```python
from build123d import *

# Parameters (mm, degrees)
F1_DEPTH     = 37.30625
F2_DEPTH     = 15.875
F3_R         = 15.87499
F0_R         = 13.890625
F0_R_2       = 7.14375
F4_DEPTH     = 37.30625
F6_DEPTH     = 3.175
F7_DEPTH     = 27.78125
F8_T4_DEPTH  = 515.4304915521
F8_T9_DEPTH  = 515.4304915521
F8_T14_DEPTH = 515.4304915521
F8_T19_DEPTH = 515.4304915521
F8_T24_DEPTH = 515.4304915521
F8_T29_DEPTH = 515.4304915521
F9_DEPTH     = 50.8
F10_R        = 6.35
F11_DEPTH    = 14.5721768419
F12_DEPTH    = 38.1


# Not quite as in the source:
# - a fillet or chamfer that OpenCascade refuses, or shapes differently, is made with other operations: its cross-section is extruded or revolved along the edge and cut away or added
# - a fillet or chamfer is up to 0.001 mm smaller than in the source, because OpenCascade refuses the exact size
# - a feature of the source that left no trace in its solid (it failed there, or was rolled back) is left out


with BuildPart() as f1:
    # F0 (on Front) → F1 (new body, symmetric)
    with BuildSketch(Plane.XZ):
        with BuildLine():
            Line((15.875, 0), (27.78125, 0))
            ThreePointArc((27.78125, 0), (26.7293483379, 7.5723040742), (23.6533011862, 14.5711768419))
            ThreePointArc((23.6533011862, 14.5711768419), (0, 27.78125), (-23.6533011862, 14.5711768419))
            ThreePointArc((-23.6533011862, 14.5711768419), (-26.7293483379, 7.5723040742), (-27.78125, 0))
            Line((-27.78125, 0), (-15.875, 0))
            ThreePointArc((-15.875, 0), (0, 15.875), (15.875, 0))
        make_face()
    extrude(amount=F1_DEPTH, both=True)

    # F0 (on Front) → F2 (join, symmetric)
    with BuildSketch(Plane.XZ):
        with BuildLine():
            ThreePointArc((23.6533011862, 14.5711768419), (26.7293483379, 7.5723040742), (27.78125, 0))
            Line((27.78125, 0), (53.975, 0))
            Line((53.975, 0), (53.975, 14.5711768419))
            Line((53.975, 14.5711768419), (23.6533011862, 14.5711768419))
        make_face()
        with BuildLine():
            ThreePointArc((-27.78125, 0), (-26.7293483379, 7.5723040742), (-23.6533011862, 14.5711768419))
            Line((-23.6533011862, 14.5711768419), (-53.975, 14.5711768419))
            Line((-53.975, 14.5711768419), (-53.975, 0))
            Line((-53.975, 0), (-27.78125, 0))
        make_face()
    extrude(amount=F2_DEPTH, both=True)

    # F3 (radius 15.875 in the source; OpenCascade refuses exactly that, so slightly less here)
    f3_edges = [f1.edges().sort_by_distance(p)[0] for p in [
        (53.975, -15.875, 7.285588),
        (53.975, 15.875, 7.285588),
        (-53.975, -15.875, 7.285588),
        (-53.975, 15.875, 7.285588),
    ]]
    fillet(f3_edges, radius=F3_R)



with BuildPart() as f4:
    # F0 (on Front) → F4 (new body, symmetric)
    with BuildSketch(Plane.XZ):
        with Locations((0, 99.21875)):
            Circle(F0_R)
        with Locations((0, 99.21875)):
            Circle(F0_R_2, mode=Mode.SUBTRACT)
    extrude(amount=F4_DEPTH, both=True)


with BuildPart() as f1_1:
    add(f1.part)

    add(f4.part)  # F6 merges F4
    # F5 (on Right) → F6 (join, symmetric)
    with BuildSketch(Plane.YZ):
        Polygon((-15.1982219998, 89.4941017032), (-23.1018472504, 25.1242396258), (23.1018472504, 25.1242396258), (15.1982219998, 89.4941017032), align=None)
        Polygon((-9.2232641814, 73.025), (9.2232641814, 73.025), (13.8038957065, 35.71875), (-13.8038957065, 35.71875), align=None, mode=Mode.SUBTRACT)
    extrude(amount=F6_DEPTH, both=True)

    # F5 (on Right) → F7 (join, symmetric)
    with BuildSketch(Plane.YZ):
        Polygon((-21.7467648383, 100.80625), (-33.734375, 3.175), (-25.796875, 3.175), (-23.1018472504, 25.1242396258), (-15.1982219998, 89.4941017032), (-13.8092648383, 100.80625), align=None)
        Polygon((15.1982219998, 89.4941017032), (23.1018472504, 25.1242396258), (25.796875, 3.175), (33.734375, 3.175), (21.7467648383, 100.80625), (13.8092648383, 100.80625), align=None)
    extrude(amount=F7_DEPTH, both=True)

    # F8: chamfer of 13.9762738 x 97.63125 on 2 edges, made by hand


with BuildPart() as f8_tool2:
    # F8_s3 → F8_t4 (new body)
    with BuildSketch(Plane.XZ.offset(-275.4932606144)):
        Polygon((13.8049762, 100.80625), (27.78125, 3.175), (27.78125, 100.80625), align=None)
    extrude(amount=F8_T4_DEPTH)

    split(bisect_by=Plane.XY.offset(14.5711768419), keep=Keep.TOP)


with BuildPart() as f1_2:
    add(f1_1.part)

    # F8_t1: cut F8_tool2
    add(f8_tool2.part, mode=Mode.SUBTRACT)


with BuildPart() as f8_tool7:
    # F8_s8 → F8_t9 (new body)
    with BuildSketch(Plane.XZ.offset(-275.4932606144)):
        Polygon((13.8049762, 100.80625), (27.78125, 3.175), (27.78125, 100.80625), align=None)
    extrude(amount=F8_T9_DEPTH)

    split(bisect_by=Plane.XZ.offset(-15.875), keep=Keep.BOTTOM)


with BuildPart() as f1_3:
    add(f1_2.part)

    # F8_t6: cut F8_tool7
    add(f8_tool7.part, mode=Mode.SUBTRACT)


with BuildPart() as f8_tool12:
    # F8_s13 → F8_t14 (new body)
    with BuildSketch(Plane.XZ.offset(-275.4932606144)):
        Polygon((13.8049762, 100.80625), (27.78125, 3.175), (27.78125, 100.80625), align=None)
    extrude(amount=F8_T14_DEPTH)

    split(bisect_by=Plane.XZ.offset(15.875), keep=Keep.TOP)


with BuildPart() as f1_4:
    add(f1_3.part)

    # F8_t11: cut F8_tool12
    add(f8_tool12.part, mode=Mode.SUBTRACT)


with BuildPart() as f8_tool17:
    # F8_s18 → F8_t19 (new body)
    with BuildSketch(Plane.XZ.offset(-239.9372309377)):
        Polygon((-13.8049762, 100.80625), (-27.78125, 3.175), (-27.78125, 100.80625), align=None)
    extrude(amount=F8_T19_DEPTH)

    split(bisect_by=Plane.XY.offset(14.5711768419), keep=Keep.TOP)


with BuildPart() as f1_5:
    add(f1_4.part)

    # F8_t16: cut F8_tool17
    add(f8_tool17.part, mode=Mode.SUBTRACT)


with BuildPart() as f8_tool22:
    # F8_s23 → F8_t24 (new body)
    with BuildSketch(Plane.XZ.offset(-239.9372309377)):
        Polygon((-13.8049762, 100.80625), (-27.78125, 3.175), (-27.78125, 100.80625), align=None)
    extrude(amount=F8_T24_DEPTH)

    split(bisect_by=Plane.XZ.offset(-15.875), keep=Keep.BOTTOM)


with BuildPart() as f1_6:
    add(f1_5.part)

    # F8_t21: cut F8_tool22
    add(f8_tool22.part, mode=Mode.SUBTRACT)


with BuildPart() as f8_tool27:
    # F8_s28 → F8_t29 (new body)
    with BuildSketch(Plane.XZ.offset(-239.9372309377)):
        Polygon((-13.8049762, 100.80625), (-27.78125, 3.175), (-27.78125, 100.80625), align=None)
    extrude(amount=F8_T29_DEPTH)

    split(bisect_by=Plane.XZ.offset(15.875), keep=Keep.TOP)


with BuildPart() as f1_7:
    add(f1_6.part)

    # F8_t26: cut F8_tool27
    add(f8_tool27.part, mode=Mode.SUBTRACT)

    # F0 (on Front) → F9 (cut, symmetric)
    with BuildSketch(Plane.XZ):
        with BuildLine():
            Line((-15.875, 0), (15.875, 0))
            ThreePointArc((15.875, 0), (0, 15.875), (-15.875, 0))
        make_face()
    extrude(amount=F9_DEPTH, both=True, mode=Mode.SUBTRACT)

    # F10 (on face) → F11 (cut, through all)
    with BuildSketch(Plane.XY.offset(14.5711768419)):
        with Locations((-38.1, 0)):
            Circle(F10_R)
        with Locations((38.1, 0)):
            Circle(F10_R)
    extrude(amount=-F11_DEPTH, mode=Mode.SUBTRACT)

    # F0 (on Front) → F12 (cut, symmetric)
    with BuildSketch(Plane.XZ):
        with Locations((0, 99.21875)):
            Circle(F0_R_2)
    extrude(amount=F12_DEPTH, both=True, mode=Mode.SUBTRACT)


solid = f1_7.part
```
For this review, take the finished solid that the model builds, in its own axes (mm). A direction names the side the tool comes from. Give positions to 0.01 mm unless a question says otherwise; leave off trailing zeros. Order: outer loops, then holes, each group sorted by start corner. A loop starts at its lowest first (then second) coordinate and runs counter-clockwise, first axis right, second up.
1) Take a section at B-B (y = -11). State how many separate pieces and enclosed holes the cut face has, then the cut area to 3 significant figures.
2) Take a section at D-D (x = -35). Give the boundary of the cut face in (y, z) (3 decimals).
3) Wall thickness on line 1 (Z direction, x = 0, y = -0.5) (1 decimal); line 2 (X direction, y = -28, z = 99); line 3 (Z direction, x = -6, y = -7): over which ranges is each line inside the solid? List them lowest first.
4) Insertion check: pin 1 (9 mm diameter, centred on x = -40.5, y = -3.5, fed in from +Z); pin 2 (3 mm diameter, centred on x = -8.5, y = -2.5, fed in from -Z); pin 3 (12 mm diameter, centred on y = 0, z = 101.5, fed in from -X); pin 4 (7.5 mm diameter, centred on x = -38.1, y = 0, fed in from -Z). Each pin has a flat end and moves straight along its axis. Give the tip position at first contact, or say it passes through.
5) Take a section at A-A (x = 0). Give the boundary of the cut face in (y, z) (1 decimal), then the cut area to 3 significant figures.
6) The part is to be moulded in two halves that separate along Z. For faces 4 (the face through (-12.916, -19.887, 51.307)), 5 (the face through (20.695, -23.632, 52.674)), 6 (the face through (31.756, 0.279, 7.388)), say which applies: released by +Z, released by -Z, zero draft, split by the parting line, or undercut.
7) Take a section at C-C (z = 103). Give the boundary of the cut face in (x, y).
8) For faces 1 (the face through (-20.695, -23.632, 52.674)), 2 (the face through (0.04, 11.48, 54.63)), 3 (the face through (32, -3, 14.571)), list the 3-axis set-ups (+Z, -Z, +X, -X, +Y, -Y) from which the entire face can be reached by the end or side of a thin tool; tool diameter is ignored.
Derived:
1. separate pieces: 2
1. enclosed holes: 1
1. area: 2,160 mm2
2. outline: (-15.875, 0) - (-5.542, 0) - (-5.542, 14.571) - (-15.875, 14.571) - close; (5.542, 0) - (15.875, 0) - (15.875, 14.571) - (5.542, 14.571) - close
3. line 1: z = 15.9 to 35.7, 73 to 92.1, 106.4 to 113.1
3. line 2: x = -13.89 to -7.14, 7.14 to 13.89
3. line 3: z = 14.7 to 27.13, 86.69 to 95.34, 103.1 to 111.75
4. pin 1: stops at z = 14.57
4. pin 2: stops at z = 12.33
4. pin 3: stops at x = -13.89
4. pin 4: passes through
5. outline: (-37.3, 15.9) - (37.3, 15.9) - (37.3, 27.8) - (30.7, 27.8) - (23.6, 85.3) - (37.3, 85.3) - (37.3, 92.1) - (-37.3, 92.1) - (-37.3, 85.3) - (-23.6, 85.3) - (-30.7, 27.8) - (-37.3, 27.8) - close; (-37.3, 106.4) - (37.3, 106.4) - (37.3, 113.1) - (-37.3, 113.1) - close; hole (-13.8, 35.7) - (13.8, 35.7) - (9.2, 73) - (-9.2, 73) - close
5. area: 4,160 mm2
6. face 4: undercut
6. face 5: released by +Z
6. face 6: zero draft
7. outline: (-13.37, -37.31) - (-6.06, -37.31) - (-6.06, 37.31) - (-13.37, 37.31) - close; (6.06, -37.31) - (13.37, -37.31) - (13.37, 37.31) - (6.06, 37.31) - close
8. face 1: +Z, -X, -Y
8. face 2: +X, -X
8. face 3: +Z, +X
